Read the model definition and answer for the solid it produces. Units are mm, in the model's axes. Give positions to 0.01 mm unless a question says otherwise; leave off trailing zeros. Write item = value, one per line.
from build123d import *

# Parameters (mm, degrees)
SKETCH1_R           = 96.5
BOSS_EXTRUDE1_DEPTH = 3
SKETCH2_R           = 6
CUT_EXTRUDE3_DEPTH  = 10
CHAMFER3_SIZE       = 1.5


with BuildPart() as part:
    # Sketch1 → Boss-Extrude1 (new body)
    with BuildSketch(Plane(origin=(0, 0, 0), x_dir=(1, 0, 0), z_dir=(0, 1, 0))):
        with Locations(Location((0, 0, 0), (0, 0, 270))):
            Circle(SKETCH1_R)
    extrude(amount=BOSS_EXTRUDE1_DEPTH)

    # Sketch2 → Cut-Extrude3 (cut)
    with BuildSketch(Plane(origin=(0, 3, 0), x_dir=(1, 0, 0), z_dir=(0, 1, 0))):
        with Locations(Location((30, 0, 0), (0, 0, 270))):
            Circle(SKETCH2_R)
        with Locations(Location((53.125920446, 14.235047481, 0), (0, 0, 270))):
            Circle(SKETCH2_R)
        with Locations(Location((78.784620241, 13.891854213, 0), (0, 0, 270))):
            Circle(SKETCH2_R)
        with Locations(Location((15, -25.980762114, 0), (0, 0, 270))):
            Circle(SKETCH2_R)
        with Locations(Location((-15, -25.980762114, 0), (0, 0, 270))):
            Circle(SKETCH2_R)
        with Locations(Location((-30, 0, 0), (0, 0, 270))):
            Circle(SKETCH2_R)
        with Locations(Location((-15, 25.980762114, 0), (0, 0, 270))):
            Circle(SKETCH2_R)
        with Locations(Location((15, 25.980762114, 0), (0, 0, 270))):
            Circle(SKETCH2_R)
        with Locations(Location((53.125920446, -14.235047481, 0), (0, 0, 270))):
            Circle(SKETCH2_R)
        with Locations(Location((38.890872965, -38.890872965, 0), (0, 0, 270))):
            Circle(SKETCH2_R)
        with Locations(Location((14.235047481, -53.125920446, 0), (0, 0, 270))):
            Circle(SKETCH2_R)
        with Locations(Location((-14.235047481, -53.125920446, 0), (0, 0, 270))):
            Circle(SKETCH2_R)
        with Locations(Location((-38.890872965, -38.890872965, 0), (0, 0, 270))):
            Circle(SKETCH2_R)
        with Locations(Location((-53.125920446, -14.235047481, 0), (0, 0, 270))):
            Circle(SKETCH2_R)
        with Locations(Location((-53.125920446, 14.235047481, 0), (0, 0, 270))):
            Circle(SKETCH2_R)
        with Locations(Location((-38.890872965, 38.890872965, 0), (0, 0, 270))):
            Circle(SKETCH2_R)
        with Locations(Location((-14.235047481, 53.125920446, 0), (0, 0, 270))):
            Circle(SKETCH2_R)
        with Locations(Location((14.235047481, 53.125920446, 0), (0, 0, 270))):
            Circle(SKETCH2_R)
        with Locations(Location((38.890872965, 38.890872965, 0), (0, 0, 270))):
            Circle(SKETCH2_R)
        with Locations(Location((78.784620241, -13.891854213, 0), (0, 0, 270))):
            Circle(SKETCH2_R)
        with Locations(Location((69.282032303, -40, 0), (0, 0, 270))):
            Circle(SKETCH2_R)
        with Locations(Location((51.423008775, -61.28355545, 0), (0, 0, 270))):
            Circle(SKETCH2_R)
        with Locations(Location((27.361611466, -75.175409663, 0), (0, 0, 270))):
            Circle(SKETCH2_R)
        with Locations(Location((0, -80, 0), (0, 0, 270))):
            Circle(SKETCH2_R)
        with Locations(Location((-27.361611466, -75.175409663, 0), (0, 0, 270))):
            Circle(SKETCH2_R)
        with Locations(Location((-51.423008775, -61.28355545, 0), (0, 0, 270))):
            Circle(SKETCH2_R)
        with Locations(Location((-69.282032303, -40, 0), (0, 0, 270))):
            Circle(SKETCH2_R)
        with Locations(Location((-78.784620241, -13.891854213, 0), (0, 0, 270))):
            Circle(SKETCH2_R)
        with Locations(Location((-78.784620241, 13.891854213, 0), (0, 0, 270))):
            Circle(SKETCH2_R)
        with Locations(Location((-69.282032303, 40, 0), (0, 0, 270))):
            Circle(SKETCH2_R)
        with Locations(Location((-51.423008775, 61.28355545, 0), (0, 0, 270))):
            Circle(SKETCH2_R)
        with Locations(Location((-27.361611466, 75.175409663, 0), (0, 0, 270))):
            Circle(SKETCH2_R)
        with Locations(Location((0, 80, 0), (0, 0, 270))):
            Circle(SKETCH2_R)
        with Locations(Location((27.361611466, 75.175409663, 0), (0, 0, 270))):
            Circle(SKETCH2_R)
        with Locations(Location((51.423008775, 61.28355545, 0), (0, 0, 270))):
            Circle(SKETCH2_R)
        with Locations(Location((69.282032303, 40, 0), (0, 0, 270))):
            Circle(SKETCH2_R)
    extrude(amount=-CUT_EXTRUDE3_DEPTH, mode=Mode.SUBTRACT)

    # Chamfer3
    chamfer3_edges = [part.edges().sort_by_distance(p)[0] for p in [
        (-15, 3, -31.980762114),
        (-30, 3, -6),
        (-15, 3, 19.980762114),
        (15, 3, 19.980762114),
        (78.784620241, 3, -19.891854213),
        (53.125920446, 3, -20.235047481),
        (38.890872965, 3, 32.890872965),
        (14.235047481, 3, 47.125920446),
        (-14.235047481, 3, 47.125920446),
        (-38.890872965, 3, 32.890872965),
        (-53.125920446, 3, 8.235047481),
        (-53.125920446, 3, -20.235047481),
        (-38.890872965, 3, -44.890872965),
        (-14.235047481, 0, -59.125920446),
        (-14.235047481, 3, -59.125920446),
        (27.361611466, 3, -81.175409663),
        (51.423008775, 3, -67.28355545),
        (69.282032303, 3, -46),
        (30, 3, -6),
        (14.235047481, 0, -59.125920446),
        (14.235047481, 3, -59.125920446),
        (38.890872965, 3, -44.890872965),
        (78.784620241, 3, 7.891854213),
        (69.282032303, 3, 34),
        (51.423008775, 3, 55.28355545),
        (27.361611466, 3, 69.175409663),
        (0, 3, 74),
        (-27.361611466, 3, 69.175409663),
        (-51.423008775, 3, 55.28355545),
        (-69.282032303, 3, 34),
        (-78.784620241, 3, 7.891854213),
        (-78.784620241, 3, -19.891854213),
        (-69.282032303, 3, -46),
        (-51.423008775, 3, -67.28355545),
        (-27.361611466, 3, -81.175409663),
        (0, 3, -86),
        (53.125920446, 3, 8.235047481),
        (15, 3, -31.980762114),
    ]]
    chamfer(chamfer3_edges, length=CHAMFER3_SIZE - 0.0001)  # a hair under: the kernel refuses the full size


solid = part.part
(1) Consider L1, parallel to Z at x = 12.5, y = 2.1; L2, parallel to X at y = 0.8, z = -80; L3, parallel to X at y = 1.5, z = 28. Determine where each line is inside the solid, lowest interval first.
Checks:
L1 = -95.69 to -59.49, -46.76 to -32.09, -19.87 to 19.87, 32.09 to 46.76, 59.49 to 95.69
L2 = -53.97 to -30.93, -23.79 to -6, 6 to 23.79, 30.93 to 53.97
L3 = -92.35 to -20.65, -9.35 to 9.35, 20.65 to 92.35
(2) Given P1, Ø14, axis at x = -15, z = -25.98, coming from the +Y side; P2, Ø7, axis at x = 78.78, z = 13.89, coming from the -Y side; P3, Ø19, axis at x = 38.89, z = -38.89, coming from the -Y side, each flat-ended and moving along its own axis, determine where each tip first touches the part or whether it passes through.
Checks:
P1 = 2.5
P2 = through
P3 = 0
(3) The part is cut by section A-A on z = -25. Count the separate pieces of the cut face and the enclosed holes in it, plus the area to 3 significant figures.
Checks:
separate_pieces = 3
enclosed_holes = 0
area = 484 mm²
